For this review, take the finished solid that the model builds, in its own axes (mm). A direction names the side the tool comes from. Give positions to 0.01 mm unless a question says otherwise; leave off trailing zeros. Order: outer loops, then holes, each group sorted by start corner. A loop starts at its lowest first (then second) coordinate and runs counter-clockwise, first axis right, second up. Notation, with made-up numbers: (-40, -36.75) -> (-21, -36.75) arc R31 cw to (-21, -4.75) -> close; hole circle Ø9 at (50, 31). An arc over 180 degrees is marked (long way). Use CSV: the item, a comma, the result in double quotes. Start each with the question number.
Autodesk Inventor part; units mm, degrees
ref_plane "YZ Plane" through (0, 0, 0) normal (1, 0, 0) x (0, 1, 0)
ref_plane "XZ Plane" through (0, 0, 0) normal (0, 1, 0) x (-1, 0, 0)
ref_plane "XY Plane" through (0, 0, 0) normal (0, 0, 1) x (1, 0, 0)
sketch "Sketch1" plane through (0, 0, 0) normal (0, 1, 0) x (-1, 0, 0)
  line L0 (0, 0) -> (-160, 0)
  line L1 (-160, 0) -> (-160, -160)
  line L2 (-160, -160) -> (0, -160)
  line L3 (0, -160) -> (0, 0)
  dimension "d0" = 160
  dimension "d1" = 160
extrude "Extrusion1" add sketch "Sketch1" along normal blind 14
sketch "Sketch2" plane through (0, 14, 0) normal (0, 1, 0) x (1, 0, 0)
  line L0 (54.75, 30) -> (105.25, 30)
  line L1 (105.25, 30) -> (105.25, 56.5)
  line L2 (105.25, 56.5) -> (54.75, 56.5)
  line L3 (54.75, 56.5) -> (54.75, 30)
  line L4 (0, 0) -> (160, 0)
  line L5 (0, 160) -> (0, 0)
  line L6 (11.0918, 136.251) -> (15.6934, 110.1536)
  line L7 (15.6934, 110.1536) -> (65.4262, 118.9228)
  line L8 (65.4262, 118.9228) -> (60.8246, 145.0203)
  line L9 (60.8246, 145.0203) -> (11.0918, 136.251)
  line L10 (38.2588, 94.75) -> (38.2588, 145.25) construction
  line L11 (25.009, 127.5869) -> (51.509, 127.5869) construction
  line L12 (160, 160) -> (0, 160)
  line L13 (54.75, 43.25) -> (106.8484, 43.25) construction
  line L14 (80, 30) -> (80, 56.5) construction
  line L15 (80, 43.25) -> (80, 148.25)
  line L16 (148.9082, 136.251) -> (144.3066, 110.1536)
  line L17 (144.3066, 110.1536) -> (94.5738, 118.9228)
  line L18 (94.5738, 118.9228) -> (99.1754, 145.0203)
  line L19 (99.1754, 145.0203) -> (148.9082, 136.251)
  line L20 (98.0138, 136.2229) -> (145.4682, 118.9509) construction
  line L21 (126.2728, 140.0379) -> (117.2092, 115.136) construction
  line L22 (121.741, 127.5869) -> (85.8289, 28.9192)
  line L23 (38.259, 127.5869) -> (56.4995, 24.14) construction
  point P0 (38.2588, 120)
  point P1 (33.7272, 140.0379)
  point P2 (61.9862, 136.2229)
  dimension "d4" = 26.5
  dimension "d5" = 50.5
  dimension "d6" = 30
  dimension "d7" = 80
  dimension "d9" = 27.167
  dimension "d13" = 17.4333
  dimension "d15" = 12.4509
  dimension "d16" = 23.7272
  dimension "d17" = 11.0918
  dimension "d19" = 105
  dimension "d73" = 270
extrude "Extrusion2" cut sketch "Sketch2" against normal blind 7
sketch "Sketch3" plane through (0, 7, 0) normal (0, 1, 0) x (1, 0, 0)
  circle A0 centre (21.1254, 118.2194) radius 1.8
  line L0 (11.0918, 136.251) -> (60.8246, 145.0203) construction
  line L1 (35.9582, 140.6356) -> (40.5598, 114.5382) construction
  line L2 (65.4262, 118.9228) -> (15.6934, 110.1536) construction
  circle A1 centre (18.9548, 130.5295) radius 1.8
  line L3 (15.6934, 110.1536) -> (11.0918, 136.251)
  circle A2 centre (57.5633, 124.6444) radius 1.8
  circle A3 centre (55.3926, 136.9545) radius 1.8
  line L4 (160, 160) -> (0, 160) construction
  line L5 (80, 160) -> (80, 0) construction
  line L6 (0, 0) -> (160, 0) construction
  circle A4 centre (138.8746, 118.2194) radius 1.8
  line L7 (124.0418, 140.6356) -> (119.4402, 114.5382) construction
  circle A5 centre (141.0452, 130.5295) radius 1.8
  circle A6 centre (102.4367, 124.6444) radius 1.8
  circle A7 centre (104.6074, 136.9545) radius 1.8
  circle A8 centre (61.5, 37) radius 1.8
  circle A9 centre (61.5, 49.5) radius 1.8
  line L8 (54.75, 56.5) -> (105.25, 56.5)
  line L9 (54.75, 30) -> (54.75, 56.5)
  line L10 (105.25, 30) -> (54.75, 30)
  circle A10 centre (98.5, 37) radius 1.8
  circle A11 centre (98.5, 49.5) radius 1.8
  circle A12 centre (120.6123, 121.1857) radius 1
  line L11 (144.3066, 110.1536) -> (94.5738, 118.9228)
  circle A13 centre (127.4464, 131.1503) radius 1.25
  line L12 (148.9082, 136.251) -> (144.3066, 110.1536)
  line L13 (127.4464, 131.1503) -> (129.9085, 130.7162) construction
  line L14 (129.9085, 130.7162) -> (124.9844, 131.5845) construction
  line L15 (99.1754, 145.0203) -> (148.9082, 136.251) construction
  arc A14 (129.9085, 130.7162) -> (124.9844, 131.5845) centre (127.1209, 129.3038) ccw
  arc A15 (124.9844, 131.5845) -> (129.9085, 130.7162) centre (127.772, 132.9968) ccw
  circle A16 centre (117.5984, 132.8868) radius 1.25
  line L16 (117.5984, 132.8868) -> (115.1364, 133.3209) construction
  line L17 (115.1364, 133.3209) -> (120.0604, 132.4527) construction
  arc A17 (120.0604, 132.4527) -> (115.1364, 133.3209) centre (117.2728, 131.0403) ccw
  arc A18 (115.1364, 133.3209) -> (120.0604, 132.4527) centre (117.924, 134.7333) ccw
  circle A19 centre (39.3877, 121.1857) radius 1
  circle A20 centre (32.5536, 131.1503) radius 1.25
  line L18 (32.5536, 131.1503) -> (30.0915, 130.7162) construction
  line L19 (30.0915, 130.7162) -> (35.0156, 131.5845) construction
  arc A21 (35.0156, 131.5845) -> (30.0915, 130.7162) centre (32.8791, 129.3038) ccw
  arc A22 (30.0915, 130.7162) -> (35.0156, 131.5845) centre (32.228, 132.9968) ccw
  line L20 (42.4016, 132.8868) -> (44.8636, 133.3209) construction
  circle A23 centre (42.4016, 132.8868) radius 1.25
  line L21 (44.8636, 133.3209) -> (39.9396, 132.4527) construction
  arc A24 (39.9396, 132.4527) -> (44.8636, 133.3209) centre (42.076, 134.7333) ccw
  arc A25 (44.8636, 133.3209) -> (39.9396, 132.4527) centre (42.7272, 131.0403) ccw
  circle A26 centre (80, 49.75) radius 1
  circle A27 centre (85, 38.75) radius 1.25
  line L22 (105.25, 56.5) -> (105.25, 30)
  line L23 (85, 38.75) -> (87.5, 38.75) construction
  line L24 (87.5, 38.75) -> (82.5, 38.75) construction
  arc A28 (82.5, 38.75) -> (87.5, 38.75) centre (85, 40.625) ccw
  arc A29 (87.5, 38.75) -> (82.5, 38.75) centre (85, 36.875) ccw
  circle A30 centre (75, 38.75) radius 1.25
  line L25 (75, 38.75) -> (72.5, 38.75) construction
  line L26 (72.5, 38.75) -> (77.5, 38.75) construction
  arc A31 (72.5, 38.75) -> (77.5, 38.75) centre (75, 40.625) ccw
  arc A32 (77.5, 38.75) -> (72.5, 38.75) centre (75, 36.875) ccw
  line L27 (54.75, 43.25) -> (105.25, 43.25) construction
  line L28 (105.25, 56.5) -> (105.25, 30) construction
  line L29 (146.6074, 123.2023) -> (96.8746, 131.9716) construction
  line L30 (94.5738, 118.9228) -> (99.1754, 145.0203) construction
  point P0 (80, 59.75)
  point P1 (80, 69.75)
  point P2 (127.4464, 131.1503)
  dimension "d24" = 3.6
  dimension "d25" = 7
  dimension "d26" = 6.75
  dimension "d27" = 6.75
  dimension "d28" = 7
  dimension "d29" = 7
  dimension "d30" = 6.75
  dimension "d31" = 3.6
  dimension "d32" = 6.75
  dimension "d33" = 7
  dimension "d36" = 2
  dimension "d37" = 6.75
  dimension "d38" = 2.5
  dimension "d39" = 20.25
  dimension "d41" = 2.5
  dimension "d42" = 2.5
  dimension "d43" = 2
  dimension "d44" = 6.75
  dimension "d45" = 2.5
  dimension "d46" = 20.25
  dimension "d48" = 2.5
  dimension "d49" = 2.5
  dimension "d74" = 10
  dimension "d75" = 10
  dimension "d79" = 4.5
  dimension "d80" = 4.5
extrude "Extrusion3" cut sketch "Sketch3" against normal blind 7 contours A0 | A1 | A2 | A3 | A4 | A5 | A6 | A7 | A8 | A9 | A10 | A11 | A12 | A13 | A13 A14 A15 | A13 A15 A14 | A16 | A16 A17 A18 | A16 A18 A17 | A19 | A20 | A20 A21 A22 | A20 A22 A21 | A23 | A23 A25 A24 | A23 A24 A25 | A26 | A27 | A27 A29 A28 | A27 A28 A29 | A30 | A30 A32 A31 | A30 A31 A32
sketch "Sketch5" plane through (0, 14, 0) normal (0, 1, 0) x (1, 0, 0)
  line L0 (0, 160) -> (0, 0)
  line L1 (0, 144.4495) -> (88.1912, 160)
  line L2 (160, 160) -> (0, 160)
  line L3 (71.8088, 160) -> (160, 144.4495)
  line L4 (160, 0) -> (160, 160)
  line L5 (11.0918, 136.251) -> (60.8246, 145.0203)
  line L6 (99.1754, 145.0203) -> (148.9082, 136.251)
  line L7 (0, 120) -> (59.75, 0)
  line L8 (0, 0) -> (160, 0)
  line L9 (160, 120) -> (100.25, 0)
  line L10 (54.75, 30) -> (54.75, 56.5)
  line L11 (105.25, 56.5) -> (105.25, 30)
  line L12 (0, 144.4495) -> (0, 160)
  line L13 (88.1912, 160) -> (0, 160)
  line L14 (160, 144.4495) -> (160, 160)
  line L15 (71.8088, 160) -> (160, 160)
  line L16 (160, 0) -> (160, 120)
  line L17 (100.25, 0) -> (160, 0)
  line L18 (0, 120) -> (0, 0)
  line L19 (0, 0) -> (59.75, 0)
  line L20 (49.7917, 20) -> (110.2083, 20)
  line L21 (105.25, 30) -> (54.75, 30)
  line L22 (160, 144.4495) -> (134.5297, 0)
  line L23 (0, 0) -> (160, 0)
  line L24 (148.9082, 136.251) -> (144.3066, 110.1536)
  line L25 (0, 144.4495) -> (25.4703, 0)
  line L26 (15.6934, 110.1536) -> (11.0918, 136.251)
  line L27 (0, 160) -> (0, 0)
  line L28 (0, 155) -> (160, 155)
  point P0 (115.9044, 152.2248)
  point P1 (100.25, 0)
  point P2 (71.8088, 160)
  point P3 (153.3251, 106.5944)
  point P4 (6.6749, 106.5944)
  point P5 (59.8348, 155)
  point P6 (100.1652, 155)
  point P7 (80, 158.5557)
  dimension "d50" = 10
  dimension "d51" = 10
  dimension "d52" = 120
  dimension "d54" = 120
  dimension "d56" = 5
  dimension "d57" = 5
  dimension "d60" = 10
  dimension "d78" = 5
extrude "Extrusion4" cut sketch "Sketch5" against normal through all contours L2 L3 L1 L28 L0 | L28 L1 L0 | L2 L1 L3 | L25 L7 L0 | L1 L3 L28 | L2 L4 L28 L3 L1 | L7 L25 L8 L0 | L7 L8 L25 | L28 L4 L3 | L20 L9 L8 L7 | L4 L9 L22 | L9 L22 L8 | L4 L8 L22 L9
fillet "Fillet1" radius 12 8 edges at (110.2083, 7, -20) (49.7917, 7, -20) (0, 7, -144.4495) (6.6749, 7, -106.5944) (59.8348, 7, -155) (100.1652, 7, -155) (160, 7, -144.4495) (153.3251, 7, -106.5944)
sketch "Sketch6" plane through (0, 14, 0) normal (0, 1, 0) x (1, 0, 0)
  circle A0 centre (80, 90) radius 34
  line L0 (99.96, 160) -> (60.04, 160)
  line L1 (160, 120.9408) -> (160, 141.0931)
  line L2 (80, 90) -> (80, 18.0727) construction
  line L3 (80, 90) -> (28.0347, 59.9978) construction
  line L4 (80, 90) -> (140.0044, 90) construction
  circle A1 centre (50.5551, 73) radius 1.8
  circle A2 centre (109.4449, 73) radius 1.8
  circle A3 centre (80, 124) radius 1.8
  point P0 (0, 0)
  dimension "d62" = 68
  dimension "d63" = 70
  dimension "d64" = 80
  dimension "d65" = 150
  dimension "d66" = 3.6
  dimension "d69" = 360
extrude "Extrusion5" cut sketch "Sketch6" against normal through all contours A3 A0 | A0 A3 | A2 A0 | A0 A2 | A1 A0 | A0 A1
properties part number "Baseplate"
1. Consider section A-A (y = 8.75). State how many separate pieces and enclosed holes the cut face has, plus the area to 3 significant figures.
2. Clearance check with flat-ended pins moving along their axes: P1, Ø6, axis at x = 141.05, z = -130.53, coming from the +Y side; P2, Ø5, axis at y = 11.5, z = -64.5, coming from the -X side; P3, Ø3, axis at x = 61.5, z = -37, coming from the -Y side; P4, Ø2, axis at x = 33.5, y = 6.5, coming from the +Z side. State where each tip first meets the part, or that it passes through.
3. Consider section B-B (x = 32.5). State the section outline as (y, z) points, plus the area to 3 significant figures.
4. For faces 1 (the face through (121, 7, -128)), 2 (the face through (80, 7, -20)), 3 (the face through (75, 3.5, -37.5)), list the 3-axis set-ups (+Z, -Z, +X, -X, +Y, -Y) from which the entire face can be reached by the end or side of a thin tool; tool diameter is ignored.
5. To check wall thickness, follow L1, parallel to Z at x = 80, y = 5.75; L2, parallel to Z at x = 85, y = 0.5; L3, parallel to Z at x = 61, y = 1.5. State the ranges of each line that lie inside material, in increasing order. Write a range as [from, to].
6. Draft analysis for pull direction Z (two halves, no side actions). For faces 4 (the face through (127.189, 3.549, -129.927)), 5 (the face through (50.98, 6.9, -21.75)), 6 (the face through (34.98, 7.098, -150.617)), state which applies: +Z half, -Z half, draft (parallel to the pull), parting line (faces both ways), or undercut.
Answer list:
1,separate pieces,"1"
1,enclosed holes,"6"
1,area,"11,700 mm2"
2,P1,"y = 7"
2,P2,"x = 26.39"
2,P3,"through"
2,P4,"z = -50.71"
3,outline,"(0, -150.18) -> (14, -150.18) -> (14, -140.03) -> (7, -140.03) -> (7, -132.41) -> (0, -132.41) -> close; (0, -129.88) -> (7, -129.88) -> (7, -113.12) -> (14, -113.12) -> (14, -54.73) -> (0, -54.73) -> close"
3,area,"1,130 mm2"
4,face 1,"+Y"
4,face 2,"+Z, +X, -X, +Y, -Y"
4,face 3,"+Y, -Y"
5,L1,"[-155, -125.8], [-122.2, -50.75], [-48.75, -20]"
5,L2,"[-155, -40], [-37.5, -20]"
5,L3,"[-155, -51.23], [-47.77, -38.73], [-35.27, -20]"
6,face 4,"undercut"
6,face 5,"+Z half"
6,face 6,"-Z half"
